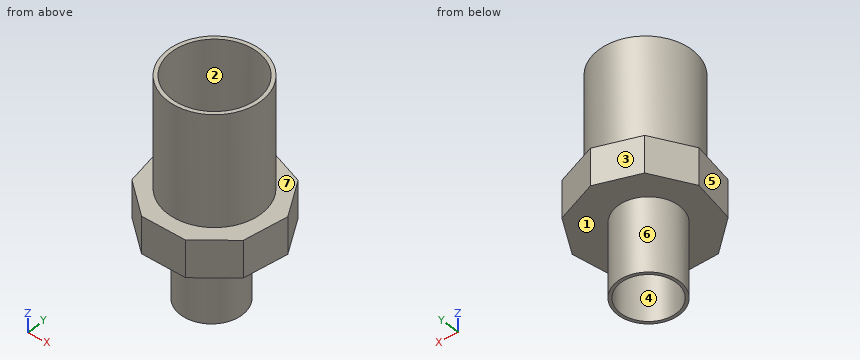
from build123d import *

# Parameters (mm, degrees)
F0_R     = 31.8925306259
F1_DEPTH = 101.6
F3_DEPTH = 25.4
F4_T     = -2.54
F5_R     = 21.061659134
F6_DEPTH = 50.8
F8_D     = 38.1


with BuildPart() as f1:
    # F0 (on Top) → F1 (new body)
    with BuildSketch(Plane.XY):
        with Locations((-10.7217477635, 10.721755214)):
            Circle(F0_R)
    extrude(amount=F1_DEPTH)

    # F2 (on Top) → F3 (join)
    with BuildSketch(Plane.XY):
        Polygon((-24.9478270625, -31.0014169663), (4.9917486821, -31.0014169663), (27.9267943106, -11.7566286384), (33.1257470788, 17.7280976768), (18.1559592065, 43.6565308501), (-9.9780391902, 53.8964688374), (-38.1120375868, 43.6565308501), (-53.0818254591, 17.7280976768), (-47.882872691, -11.7566286384), align=None)
    extrude(amount=F3_DEPTH)

    # F4
    f4_openings = [f1.faces().sort_by_distance(p)[0] for p in [
        (-10.721748, 10.721755, 101.6),
    ]]
    offset(amount=F4_T, openings=f4_openings, kind=Kind.INTERSECTION)

    # F5 (on face) → F6 (join)
    with BuildSketch(Plane(origin=(0, 0, 0), x_dir=(1, 0, 0), z_dir=(0, 0, -1))):
        with Locations((-13.595267199, -11.6091426462)):
            Circle(F5_R)
    extrude(amount=F6_DEPTH)

    # F8 (through all)
    with Locations(Plane(origin=(0, 0, -50.8), x_dir=(1, 0, 0), z_dir=(0, 0, -1))):
        with Locations((-13.595267199, -11.6091426462)):
            Hole(F8_D / 2)


solid = f1.part
Check sheet for the modelled part. Datum: model origin and axes. Units: mm. Face numbers are marked on the shaded views. A direction names the side the tool comes from. Round coordinates to 2 decimals unless told otherwise and drop trailing zeros. Loops run counter-clockwise (first coordinate to the right, second up) from the corner with the lowest first, then second, coordinate; pieces in that order, holes last. Notation, with made-up numbers: M 48,44.5 L 92,44.5 A23 cw 92,69.5 Z; hole C 32,27.25 d4. An arc over 180 degrees is marked long. One line per item, written item: value.
(1) Release check for a two-part mould opening along X. For the marked faces 1, 2, 3 and 4 record: +X half, -X half, draft (parallel to the pull), parting line (faces both ways), or undercut.
Computed values:
face 1: draft
face 2: undercut
face 3: -X half
face 4: undercut
(2) Sectioned sample at A-A, the plane z = 11. Record the cut outline in (x, y).
Computed values:
outline: M -53.08,17.73 L -47.88,-11.76 L -24.95,-31 L 4.99,-31 L 27.93,-11.76 L 33.13,17.73 L 18.16,43.66 L -9.98,53.9 L -38.11,43.66 Z; hole M -50.42,17.26 L -45.54,-10.41 L -24.02,-28.46 L 4.07,-28.46 L 25.59,-10.41 L 30.46,17.26 L 16.42,41.59 L -9.98,51.19 L -36.37,41.59 Z
(3) Sectioned sample at B-B, the plane x = 0. Record the cut outline in (y, z).
Computed values:
outline: M -31,0 L -4.48,0 L -4.48,-50.8 L -1.74,-50.8 L -1.74,2.54 L -28.46,2.54 L -28.46,22.86 L -16.6,22.86 L -16.6,101.6 L -19.31,101.6 L -19.31,25.4 L -31,25.4 Z; M 24.95,-50.8 L 27.7,-50.8 L 27.7,0 L 50.26,0 L 50.26,25.4 L 40.76,25.4 L 40.76,101.6 L 38.05,101.6 L 38.05,22.86 L 47.56,22.86 L 47.56,2.54 L 24.95,2.54 Z
(4) Sectioned sample at C-C, the plane y = 7.5. Record the cut outline in (x, z), then the cut area to 3 significant figures.
Computed values:
outline: M -51.28,0 L -34.25,0 L -34.25,-50.8 L -32.2,-50.8 L -32.2,2.54 L -48.7,2.54 L -48.7,22.86 L -39.9,22.86 L -39.9,101.6 L -42.45,101.6 L -42.45,25.4 L -51.28,25.4 Z; M 5.01,-50.8 L 7.06,-50.8 L 7.06,0 L 31.32,0 L 31.32,25.4 L 21.01,25.4 L 21.01,101.6 L 18.45,101.6 L 18.45,22.86 L 28.74,22.86 L 28.74,2.54 L 5.01,2.54 Z
area: 880 mm^2
(5) Access from +Z, -Z, +X, -X, +Y, -Y to the whole of each face (thin tool, end or side, straight path). Record for the marked faces 5, 6 and 7.
Computed values:
face 5: +Z, -Z, -X, -Y
face 6: -Z
face 7: +Z
(6) Depth check by flat-ended pin: pin 1 Ø4 at (x, y) = (-43.5, -5.5) entering from +Z; pin 2 Ø8 at (y, z) = (30, 50.5) entering from -X; pin 3 Ø24 at (x, y) = (-15, 29.5) entering from -Z; pin 4 Ø2 at (x, z) = (22.5, 40) entering from -Y. Enter the tip coordinate at first touch or a pass-through.
Computed values:
pin 1: stops at z = 25.4
pin 2: stops at x = -38.72
pin 3: stops at z = -50.8
pin 4: passes through
(7) Thickness scan on line 1 (Z direction, x = -2, y = -23.5); line 2 (Y direction, x = -12, z = 66.5); line 3 (Z direction, x = -31, y = 20.5). Record the ranges inside material, lowest first.
Computed values:
line 1: z = 0 to 2.54, 22.86 to 25.4
line 2: y = -21.15 to -18.6, 40.05 to 42.59
line 3: z = -50.8 to 2.54
(8) Sectioned sample at D-D, the plane z = -41. Record the cut outline in (x, y).
Computed values:
outline: C -13.6,11.61 d42.12; hole C -13.6,11.61 d38.1
